CAD build for the part. Positions are in the model's coordinates, mm. A direction names the side the tool comes from. Give positions to 0.01 mm unless a question says otherwise; leave off trailing zeros. Order: outer loops, then holes, each group sorted by start corner. A loop starts at its lowest first (then second) coordinate and runs counter-clockwise, first axis right, second up. Notation, with made-up numbers: M -9.75,49 L -1.75,49 A12 cw -1.75,72 Z; hole C 3,44 d11. An arc over 180 degrees is marked long. Put each result on its own line as item: value. Start each with the question number.
1) Tool access for faces 1 (the face through (-49.652, 7.276, -2.671)), 2 (the face through (6.31, 17.75, -0.55)), 3 (the face through (19.05, 1, -2)): list every direction of +Z, -Z, +X, -X, +Y, -Y with a clear straight run to the whole face (end or side of a thin tool).
2) Two-plate mould, pull along Z, no slides. Class faces 4 (the face through (35.19, -9.15, -0.4)), 5 (the face through (-1.932, 7.276, -2.671)), 6 (the face through (8, 0, -14.288)): released by +Z, released by -Z, zero draft, split by the parting line, or undercut.
3) Cut at A-A (x = -10.5). Write the cut outline in (y, z), and give its area (3 significant figures).
4) Drill centre lines: line 1 (Y direction, x = 32, z = 0); line 2 (Z direction, x = -20, y = -5); line 3 (Y direction, x = 35, z = 0). Where is each one in solid material? Low to high. Write a range as [from, to].
5) Pin check, flat tips, straight feed: pin 1 (1.5 mm diameter, centred on x = -2, z = -1.5, fed in from +Y); pin 2 (6 mm diameter, centred on x = -29, z = 0, fed in from -Y); pin 3 (10 mm diameter, centred on y = 12.5, z = 10.5, fed in from +X). Stop position of each tip, or through.
```python
from build123d import *

# Parameters (mm, degrees)
SKETCH1_R           = 19.05
EXTRUDE1_DEPTH      = 19.05
EXTRUDE1_DEPTH_BACK = 50.8
CUT_EXTRUDE1_REACH  = 52.8
SKETCH2_R           = 19.05
SKETCH2_R_2         = 13.3604
CUT_EXTRUDE3_REACH  = 21.05
SKETCH19_R          = 8.6614
CUT_EXTRUDE4_DEPTH  = 0.254
SKETCH20_R          = 8.6614
CUT_EXTRUDE5_DEPTH  = 0.254
CHAMFER1_SIZE       = 0.762
CIRPATTERN1_COUNT   = 4


with BuildPart() as part:
    # Sketch1 → Extrude1 (new body, two sides)
    with BuildSketch(Plane(origin=(0, 0, 0), x_dir=(0, 0, -1), z_dir=(1, 0, 0))) as extrude1_sk:
        Circle(SKETCH1_R)
    extrude(amount=EXTRUDE1_DEPTH)
    extrude(extrude1_sk.sketch, amount=-EXTRUDE1_DEPTH_BACK)

    # Sketch2 → Cut-Extrude1 (cut, up to next)
    with BuildSketch(Plane(origin=(0, 0, 0), x_dir=(0, 0, -1), z_dir=(1, 0, 0)), mode=Mode.PRIVATE) as cut_extrude1_sk1:
        Circle(SKETCH2_R)
        with Locations((0, -4.7498)):
            Circle(SKETCH2_R_2, mode=Mode.SUBTRACT)
    cut_extrude1_tool1 = extrude(cut_extrude1_sk1.sketch, amount=-CUT_EXTRUDE1_REACH, mode=Mode.PRIVATE) & part.part
    add(cut_extrude1_tool1.solids().sort_by_distance((0, 0, 18.511185))[0], mode=Mode.SUBTRACT)

    # Sketch4 → Cut-Extrude3 (cut, up to next)
    with BuildSketch(Plane.ZY, mode=Mode.PRIVATE) as cut_extrude3_sk1:
        with BuildLine():
            Line((14.2875, -12.600390619), (14.2875, 11.344778237))
            Line((14.2875, 11.344778237), (0, 18.007148903))
            Line((0, 18.007148903), (-14.2875, 11.344778237))
            Line((-14.2875, 11.344778237), (-14.2875, -12.600390619))
            ThreePointArc((-14.2875, -12.600390619), (0, 19.05), (14.2875, -12.600390619))
        make_face()
    cut_extrude3_tool1 = extrude(cut_extrude3_sk1.sketch, amount=-CUT_EXTRUDE3_REACH, mode=Mode.PRIVATE) & part.part
    add(cut_extrude3_tool1.solids().sort_by_distance((0, -0.627806, 14.782814))[0], mode=Mode.SUBTRACT)

    # Sketch6 → Cut-Revolve2 (revolve, cut)
    with BuildSketch(Plane.XY, mode=Mode.PRIVATE) as cut_revolve2_sk:
        Polygon((12.169188023, 18.007148903), (19.05, 3.2512), (19.05, 18.007148903), align=None)
    revolve(cut_revolve2_sk.sketch.rotate(Axis((1.987224567, -4.7498, 0), (1, 0, 0)), 270), axis=Axis((1.987224567, -4.7498, 0), (1, 0, 0)), mode=Mode.SUBTRACT)  # turned: the seam where the file's is

    # S2D0002 → Cut-Revolve3 (revolve, cut)
    with BuildSketch(Plane(origin=(6.35, 13.712414668, 8.609072086), x_dir=(0, 0.422618262, -0.906307787), z_dir=(1, 0, 0))):
        Polygon((0, 0), (4.5466, 0), (4.106586662, -2.0701), (3.4544, -2.722286662), (3.4544, -12.192), (0, -12.192), align=None)
    revolve(axis=Axis((6.35, 2.110224902, 3.198882147), (0, 0.906307787, 0.422618262)), mode=Mode.SUBTRACT)

    # Sketch19 → Cut-Extrude4 (cut)
    with BuildSketch(Plane(origin=(0, 14.790960552, 6.897138177), x_dir=(1, 0, 0), z_dir=(0, 0.906307787, 0.422618262))):
        with Locations((6.35, -2.00735222)):
            Circle(SKETCH19_R)
    extrude(amount=-CUT_EXTRUDE4_DEPTH, mode=Mode.SUBTRACT)

    # Sketch8 → Cut-Revolve4 (revolve, cut)
    with BuildSketch(Plane(origin=(6.35, 13.712414668, -8.609072086), x_dir=(0, -0.422618262, -0.906307787), z_dir=(1, 0, 0))):
        Polygon((0, 0), (4.5466, 0), (4.106586662, -2.0701), (3.4544, -2.722286662), (3.4544, -12.192), (0, -12.192), align=None)
    revolve(axis=Axis((6.35, 2.110224902, -3.198882147), (0, 0.906307787, -0.422618262)), mode=Mode.SUBTRACT)

    # Sketch20 → Cut-Extrude5 (cut)
    with BuildSketch(Plane(origin=(0, 14.790960552, -6.897138177), x_dir=(1, 0, 0), z_dir=(0, 0.906307787, -0.422618262))):
        with Locations((6.35, 2.00735222)):
            Circle(SKETCH20_R)
    extrude(amount=-CUT_EXTRUDE5_DEPTH, mode=Mode.SUBTRACT)

    # Sketch10 → Cut-Revolve6 (revolve, cut)
    with BuildSketch(Plane.XY, mode=Mode.PRIVATE) as cut_revolve6_sk:
        Polygon((0, 8.6106), (0, 7.5692), (-3.81, 7.5692), (-4.8514, 8.6106), align=None)
    revolve(cut_revolve6_sk.sketch.rotate(Axis((-5.09397, -4.7498, 0), (1, 0, 0)), 90), axis=Axis((-5.09397, -4.7498, 0), (1, 0, 0)), mode=Mode.SUBTRACT)  # turned: the seam where the file's is

    # Sketch12 → Cut-Revolve8 (revolve, cut)
    with BuildSketch(Plane.XY, mode=Mode.PRIVATE) as cut_revolve8_sk:
        Polygon((-50.8, 8.6106), (-50.8, 7.5692), (-49.276, 7.5692), (-48.2346, 8.6106), align=None)
    revolve(cut_revolve8_sk.sketch.rotate(Axis((-50.92827, -4.7498, 0), (1, 0, 0)), 90), axis=Axis((-50.92827, -4.7498, 0), (1, 0, 0)), mode=Mode.SUBTRACT)  # turned: the seam where the file's is

    # Chamfer1
    chamfer1_edges = [part.edges().sort_by_distance(p)[0] for p in [
        (-50.8, -4.7498, -12.319),
    ]]
    chamfer(chamfer1_edges, length=CHAMFER1_SIZE)

    # Sketch13 → Revolve1 (revolve)
    with BuildSketch(Plane(origin=(0, 0, 0), x_dir=(0, -1, 0), z_dir=(0, 0, 1)), mode=Mode.PRIVATE) as revolve1_sk:
        with BuildLine():
            Line((4.7498, 19.05), (4.7498, 39.3192))
            Line((4.7498, 39.3192), (9.29005, 39.3192))
            ThreePointArc((9.29005, 39.3192), (10.00847049, 39.02162049), (10.30605, 38.3032))
            Line((10.30605, 38.3032), (10.30605, 19.05))
            Line((10.30605, 19.05), (4.7498, 19.05))
        make_face()
    revolve(revolve1_sk.sketch.rotate(Axis((18.03654, -4.7498, 0), (1, 0, 0)), 270), axis=Axis((18.03654, -4.7498, 0), (1, 0, 0)))  # turned: the seam where the file's is

    # S2D0001 → Cut-Revolve9 (revolve, cut)
    with BuildSketch(Plane(origin=(39.3192, -7.5565, 0), x_dir=(0, -1, 0), z_dir=(0, 0, 1)), mode=Mode.PRIVATE) as cut_revolve9_sk:
        Polygon((0, 0), (0, -10.16), (-2.8067, -11.846435499), (-2.8067, 0), align=None)
    revolve(cut_revolve9_sk.sketch.rotate(Axis((26.880442726, -4.7498, 0), (1, 0, 0)), 270), axis=Axis((26.880442726, -4.7498, 0), (1, 0, 0)), mode=Mode.SUBTRACT)  # turned: the seam where the file's is

    # Sketch16 → Cut-Revolve10 (revolve, cut)
    with BuildSketch(Plane(origin=(35.3568, 2.197634211, 0), x_dir=(-1, 0, 0), z_dir=(0, 0, -1)), mode=Mode.PRIVATE) as cut_revolve10_sk:
        Polygon((0, -1.391184211), (1.5875, -1.391184211), (0, -2.978684211), align=None)
    cut_revolve10 = revolve(cut_revolve10_sk.sketch.rotate(Axis((35.3568, -1.281162177, 0), (0, 1, 0)), 90), axis=Axis((35.3568, -1.281162177, 0), (0, 1, 0)), mode=Mode.SUBTRACT)  # turned: the seam where the file's is

    # CirPattern1: Cut-Revolve10 ×4 about axis
    cirpattern1_axis = Axis((18.03654, -4.7498, 0), (-1, 0, 0))
    for i in range(1, CIRPATTERN1_COUNT):
        add(cut_revolve10.rotate(cirpattern1_axis, i * 360 / CIRPATTERN1_COUNT), mode=Mode.SUBTRACT)


solid = part.part
```
Solution:
1. face 1: -X
1. face 2: -Z, +X, -X, +Y
1. face 3: +X
2. face 4: undercut
2. face 5: split by the parting line
2. face 6: released by -Z
3. outline: C -4.75,0 d26.72
3. area: 561 mm²
4. line 1: [-10.31, -7.56], [-1.94, 0.81]
4. line 2: [-13.36, 13.36]
4. line 3: [-9.08, -7.56], [-1.94, -0.42]
5. pin 1: y = 7.55
5. pin 2: y = -18.11
5. pin 3: x = 15.7
